Check sheet for the modelled part. Datum: model origin and axes. Units: mm. Face numbers are marked on the shaded views. A direction names the side the tool comes from. Give positions to 0.01 mm unless a question says otherwise; leave off trailing zeros. Write each loop counter-clockwise with the first axis right and the second up, starting at its lowest first coordinate (ties: lowest second). Pieces come first, ordered by that corner, then holes.
Autodesk Inventor part; units mm, degrees
ref_plane "YZ Plane" through (0, 0, 0) normal (1, 0, 0) x (0, 1, 0)
ref_plane "XZ Plane" through (0, 0, 0) normal (0, 1, 0) x (-1, 0, 0)
ref_plane "XY Plane" through (0, 0, 0) normal (0, 0, 1) x (1, 0, 0)
sketch "Sketch1" plane through (0, 0, 0) normal (0, 0, 1) x (1, 0, 0)
  circle A0 centre (-10.16, 0) radius 2.2543
  circle A1 centre (0, 0) radius 2.2543
  circle A2 centre (10.16, 0) radius 2.2543
  line L0 (-19.05, 6.35) -> (19.05, 6.35)
  line L1 (19.05, 6.35) -> (19.05, 0)
  line L2 (19.05, 0) -> (-19.05, 0)
  line L3 (-19.05, 0) -> (-19.05, 6.35)
  dimension "d0" = 4.5085
  dimension "d3" = 10.16
  dimension "d4" = 10.16
  dimension "d5" = 6.35
  dimension "d6" = 38.1
extrude "Extrusion1" add sketch "Sketch1" along normal blind 27.94 contours L2 A0 | A0 L2 L3 L0 L1 A2 A1 | A1 L2 | A2 L2 picked at (-10.9114, 0.6984) picked at (0.5625, 0.4983) picked at (9.4728, 0.529)
extrude "Extrusion2" cut sketch "Sketch1" along normal blind 20.574 contours L2 A0 | A0 L2 | L2 A1 | A1 L2 | L2 A2 | A2 L2
sketch "Sketch2" plane through (0, 0, 27.94) normal (0, 0, 1) x (1, 0, 0)
  circle A0 centre (0, 0) radius 2.2543
  circle A1 centre (10.16, 0) radius 2.2543
  circle A2 centre (-10.16, 0) radius 2.2543
  circle A3 centre (-10.16, 0) radius 2.032
  circle A4 centre (0, 0) radius 2.032
  circle A5 centre (10.16, 0) radius 2.032
  dimension "d11" = 4.064
extrude "Extrusion3" cut sketch "Sketch2" against normal through all contours A3 | A4 | A5
sketch "Sketch3" plane through (0, 0, 0) normal (0, 1, 0) x (-1, 0, 0)
  point P0 (-16.002, 13.97)
  point P1 (0, 0)
  dimension "d38" = 13.97
  dimension "d39" = 16.002
hole "Hole1" at (16.002, 0, 13.97) direction (0, 1, 0) diameter 3.2766 end through all
mirror "Mirror1" about plane through (0, 0, 0) normal (1, 0, 0) of "Hole1"
sketch "Sketch7" plane through (0, 0, 0) normal (0, 0, 1) x (1, 0, 0)
  line L0 (-19.05, 6.35) -> (19.05, 6.35)
  line L1 (19.05, 6.35) -> (-19.05, 6.35)
  line L2 (-19.05, 6.35) -> (-19.05, 12.7)
  line L3 (-19.05, 12.7) -> (19.05, 12.7)
  line L4 (19.05, 12.7) -> (19.05, 6.35)
  point P0 (0, 10.033)
  point P1 (0, 0)
  point P2 (0, 10.033)
  dimension "d40" = 6.35
  dimension "d41" = 3.683
extrude "Extrusion5" add sketch "Sketch7" along normal blind 6.35
hole "Hole2" at (0, 10.033, 0) direction (0, 0, 1) diameter 3.2766 end through all
sketch "Sketch8" plane through (0, 0, 0) normal (0, 0, -1) x (-1, 0, 0)
  line L0 (19.05, 12.7) -> (19.05, 0)
  line L1 (-19.05, 12.7) -> (-19.05, 0)
  line L2 (-19.05, 12.7) -> (19.05, 12.7)
  line L3 (15.24, 0) -> (15.24, 16.51)
  line L4 (15.24, 16.51) -> (-22.86, 16.51)
  line L5 (-22.86, 16.51) -> (-22.86, 0)
  line L6 (-22.86, 0) -> (-19.05, 0)
  line L7 (19.05, 0) -> (15.24, 0)
  point P0 (19.05, 6.35)
  point P1 (-19.05, 6.35)
  dimension "d49" = 3.81
extrude "Extrusion6" [suppressed]
sketch "Sketch9" plane through (0, 0, 0) normal (0, 0, -1) x (-1, 0, 0)
  line L0 (19.05, 0) -> (19.05, 6.35)
  line L1 (-19.05, 6.35) -> (-19.05, 0)
  line L2 (-22.86, 0) -> (-22.86, 6.35)
  line L3 (22.86, 6.35) -> (22.86, 0)
  line L4 (-22.86, 0) -> (-19.05, 0)
  line L5 (19.05, 0) -> (22.86, 0)
  line L6 (-22.86, 6.35) -> (-19.05, 6.35)
  line L7 (19.05, 6.35) -> (22.86, 6.35)
  line L8 (-19.05, 6.35) -> (-19.05, 0)
  dimension "d48" = 3.81
extrude "Extrusion7" [suppressed]
equation "\"d49\" = FlangeWidth"
equation "\"d48\" = FlangeWidth"
equation "\"FlangeWidth\" = 3.81"
properties part number "keyhole holder-01"
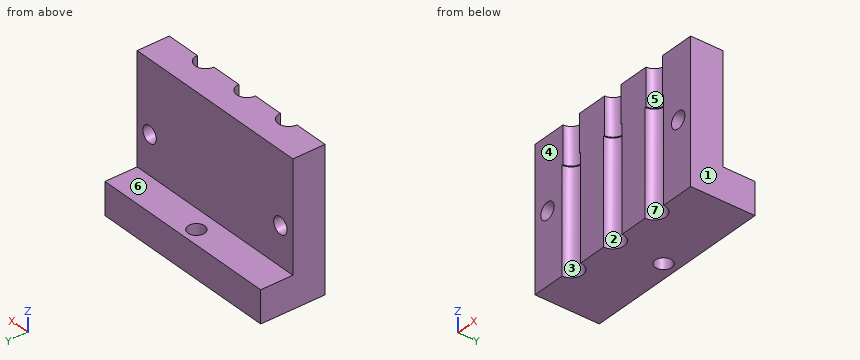
1) Sectioned sample at A-A on z = 13.97. Record the boundary of the cut face in (x, y), then the cut area to 3 significant figures.
2) Draft check along X on the marked faces 1, 2, 3 and 4. Enter one of: +X half, -X half, draft (parallel to the pull), parting line (faces both ways), or undercut.
3) Sectioned sample at C-C on z = 21.25. Record the boundary of the cut face in (x, y).
4) Access from +Z, -Z, +X, -X, +Y, -Y to the whole of each face (thin tool, end or side, straight path). Record for the marked faces 5, 6 and 7.
5) Scan lines: L1, parallel to X at y = 4, z = 13.97; L2, parallel to Z at x = -16, y = 4.5; L3, parallel to Y at x = -13.5, z = 10.25. Record each from-to range of solid material in increasing order.
6) Sectioned sample at D-D on x = -10.16. Record the boundary of the cut face in (y, z).
7) Sectioned sample at B-B on x = 0. Record the boundary of the cut face in (y, z).
8) Gauge pin test, flat ends, axial feed: pin 1 (1 mm diameter, centred on y = 7.5, z = 20.5, fed in from +X); pin 2 (4 mm diameter, centred on x = -6, z = 13.5, fed in from +Y); pin 3 (5 mm diameter, centred on x = -6, y = 9.5, fed in from +Z). Record the tip position at first contact, or that the pin passes through.
Answers below:
1. outline: (-19.05, 0) - (-17.64, 0) - (-17.64, 6.35) - (-19.05, 6.35) - close; (-14.36, 0) - (-12.41, 0) arc R2.25 cw to (-7.91, 0) - (-2.25, 0) arc R2.25 cw to (2.25, 0) - (7.91, 0) arc R2.25 cw to (12.41, 0) - (14.36, 0) - (14.36, 6.35) - (-14.36, 6.35) - close; (17.64, 0) - (19.05, 0) - (19.05, 6.35) - (17.64, 6.35) - close
1. area: 176 mm2
2. face 1: +X half
2. face 2: undercut
2. face 3: undercut
2. face 4: draft
3. outline: (-19.05, 0) - (-12.19, 0) arc R2.03 cw to (-8.13, 0) - (-2.03, 0) arc R2.03 cw to (2.03, 0) - (8.13, 0) arc R2.03 cw to (12.19, 0) - (19.05, 0) - (19.05, 6.35) - (-19.05, 6.35) - close
4. face 5: +Z, -Z, -Y
4. face 6: +Z, +X, -X, +Y
4. face 7: -Z, -Y
5. L1: x = -19.05 to -17.64, -14.36 to 14.36, 17.64 to 19.05
5. L2: z = 0 to 12.33, 15.61 to 27.94
5. L3: y = 0 to 6.35
6. outline: (2.03, 20.57) - (2.25, 20.57) - (2.25, 0) - (12.7, 0) - (12.7, 6.35) - (6.35, 6.35) - (6.35, 27.94) - (2.03, 27.94) - close
7. outline: (2.03, 20.57) - (2.25, 20.57) - (2.25, 0) - (8.39, 0) - (8.39, 6.35) - (6.35, 6.35) - (6.35, 27.94) - (2.03, 27.94) - close; (11.67, 0) - (12.7, 0) - (12.7, 6.35) - (11.67, 6.35) - close
8. pin 1: passes through
8. pin 2: stops at y = 6.35
8. pin 3: stops at z = 6.35
